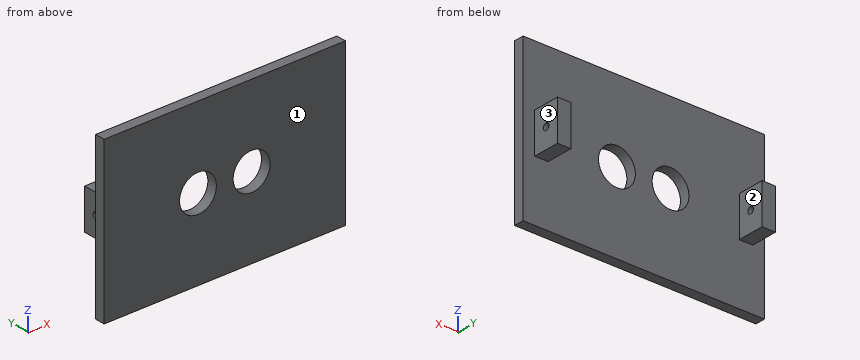
```python
from build123d import *

# Parameters (mm, degrees)
SKETCH1_W               = 114.3
SKETCH1_H               = 76.2
MAINCOVER_DEPTH         = 4.7625
SKETCH2_W               = 6.35
SKETCH2_H               = 19.05
BOSS_EXTRUDE1_DEPTH     = 12.7
SKETCH3_R               = 1.5875
CUT_EXTRUDE1_DEPTH      = 6.5245
CUT_EXTRUDE1_DEPTH_BACK = 109.7755
SKETCH4_R               = 8.73125
CUT_EXTRUDE2_DEPTH      = 18.4625


with BuildPart() as part:
    # Sketch1 → MainCover (new body)
    with BuildSketch(Plane(origin=(0, 0, 0), x_dir=(1, 0, 0), z_dir=(0, 1, 0))):
        Rectangle(SKETCH1_W, SKETCH1_H)
    extrude(amount=MAINCOVER_DEPTH)

    # Sketch2 → Boss-Extrude1 (add)
    with BuildSketch(Plane(origin=(0, 4.7625, 0), x_dir=(1, 0, 0), z_dir=(0, 1, 0))):
        with Locations((-48.4505, 0)):
            Rectangle(SKETCH2_W, SKETCH2_H)
        with Locations((48.4505, 0)):
            Rectangle(SKETCH2_W, SKETCH2_H)
    extrude(amount=BOSS_EXTRUDE1_DEPTH)

    # Sketch3 → Cut-Extrude1 (cut, two sides)
    with BuildSketch(Plane.ZY.offset(51.6255)) as cut_extrude1_sk:
        with Locations((0, 11.1125)):
            Circle(SKETCH3_R)
    extrude(amount=CUT_EXTRUDE1_DEPTH, mode=Mode.SUBTRACT)
    extrude(cut_extrude1_sk.sketch, amount=-CUT_EXTRUDE1_DEPTH_BACK, mode=Mode.SUBTRACT)

    # Sketch4 → Cut-Extrude2 (cut, through all)
    with BuildSketch(Plane.XZ):
        with Locations((12.7, 0)):
            Circle(SKETCH4_R)
        with Locations((-12.7, 0)):
            Circle(SKETCH4_R)
    extrude(amount=-CUT_EXTRUDE2_DEPTH, mode=Mode.SUBTRACT)


solid = part.part
```
Check sheet for the modelled part. Datum: model origin and axes. Units: mm. Face numbers are marked on the shaded views. Round coordinates to 2 decimals unless told otherwise and drop trailing zeros. Write each loop counter-clockwise with the first axis right and the second up, starting at its lowest first coordinate (ties: lowest second). Pieces come first, ordered by that corner, then holes. Notation, with made-up numbers: (-23, -20) -> (-14, -20) arc R24 ccw to (-14, 4) -> close; hole circle Ø3 at (-23, 5). An arc over 180 degrees is marked (long way). Put each result on its own line as item: value.
(1) Mould release check, pull along X, two halves, no side actions. Record for the marked faces 1, 2 and 3: released by +X, released by -X, zero draft, split by the parting line, or undercut.
Values found:
face 1: zero draft
face 2: undercut
face 3: released by +X
(2) Go/stop test with flat-tipped pins: pin 1 Ø6.5 at (y, z) = (10, 0) entering from +X; pin 2 Ø7 at (x, y) = (49.5, 12) entering from -Z (3 decimals); pin 3 Ø10 at (x, y) = (-22, 11) entering from +Z; pin 4 Ø3 at (x, y) = (-49.5, 11.5) entering from +Z (3 decimals). Record where each tip stops, or that it passes through.
Values found:
pin 1: stops at x = 51.63
pin 2: stops at z = -9.525
pin 3: passes through
pin 4: stops at z = 9.525
(3) Sectioned sample at D-D (x = 47). Enter the section's corners in (y, z) (1 decimal).
Values found:
outline: (0, -38.1) -> (4.8, -38.1) -> (4.8, -9.5) -> (17.5, -9.5) -> (17.5, 9.5) -> (4.8, 9.5) -> (4.8, 38.1) -> (0, 38.1) -> close; hole circle Ø3.2 at (11.1, 0)
(4) Sectioned sample at B-B (x = 12.7). Enter the section's corners in (y, z).
Values found:
outline: (0, -38.1) -> (4.76, -38.1) -> (4.76, -8.73) -> (0, -8.73) -> close; (0, 8.73) -> (4.76, 8.73) -> (4.76, 38.1) -> (0, 38.1) -> close
(5) Material ranges on line 1 (Y direction, x = -48.5, z = 0) (1 decimal); line 2 (X direction, y = 6, z = -7); line 3 (Z direction, x = 12.7, y = 3.5), recorded low to high.
Values found:
line 1: y = 0 to 9.5, 12.7 to 17.5
line 2: x = -51.63 to -45.28, 45.28 to 51.63
line 3: z = -38.1 to -8.73, 8.73 to 38.1
(6) Sectioned sample at C-C (z = 0). Count the separate pieces of the cut face and the enclosed holes in it, plus the area to 3 significant figures.
Values found:
separate pieces: 5
enclosed holes: 0
area: 499 mm^2
(7) Sectioned sample at A-A (y = 6.5). Enter the section's corners in (x, z) (1 decimal).
Values found:
outline: (-51.6, -9.5) -> (-45.3, -9.5) -> (-45.3, 9.5) -> (-51.6, 9.5) -> close; (45.3, -9.5) -> (51.6, -9.5) -> (51.6, 9.5) -> (45.3, 9.5) -> close
